Job drawing, mm, ordinate dimensions from the low corner. One solid piece. A direction names the side the tool comes from. Round coordinates to 2 decimals unless told otherwise and drop trailing zeros. Loops run counter-clockwise (first coordinate to the right, second up) from the corner with the lowest first, then second, coordinate; pieces in that order, holes last. Notation, with made-up numbers: M 70.5,69.5 L 119.5,69.5 A22 ccw 119.5,84.5 Z; hole C 63.5,19.5 d7. An arc over 180 degrees is marked long. Use a Markdown table: item, result. Add a question column.
(1) Band-saw the part on B-B, the plane z = 68. Write the cut outline in (x, y).
(2) Which spindle directions (+Z, -Z, +X, -X, +Y, -Y) get a long thin tool onto all of the face, cutting with end or side? Do the marked faces 3 and 4. Say none if no direction does.
(3) Band-saw the part on C-C, the plane x = 40. Write the cut outline in (y, z).
(4) Wall check: L1, parallel to Z at x = 75, y = 7.75; L2, parallel to X at y = 8.5, z = 6 (1 decimal). Give the ranges that are in metal, low to high.
(5) Flat gauge pins, fed straight in: P1, Ø6, axis at x = 75, z = 75, coming from the -Y side; P2, Ø1, axis at y = 3.5, z = 13, coming from the +X side (1 decimal); P3, Ø12, axis at x = 12.5, z = 29, coming from the -Y side; P4, Ø4, axis at x = 60, y = 3.5, coming from the -Z side. Where does each tip first touch, or does it go through?
(6) Two-plate mould, pull along Z, no slides. Class the marked faces 1 and 2: released by +Z, released by -Z, zero draft, split by the parting line, or undercut.
(7) Band-saw the part on A-A, the plane y = 6.75. Write the cut outline in (x, z).
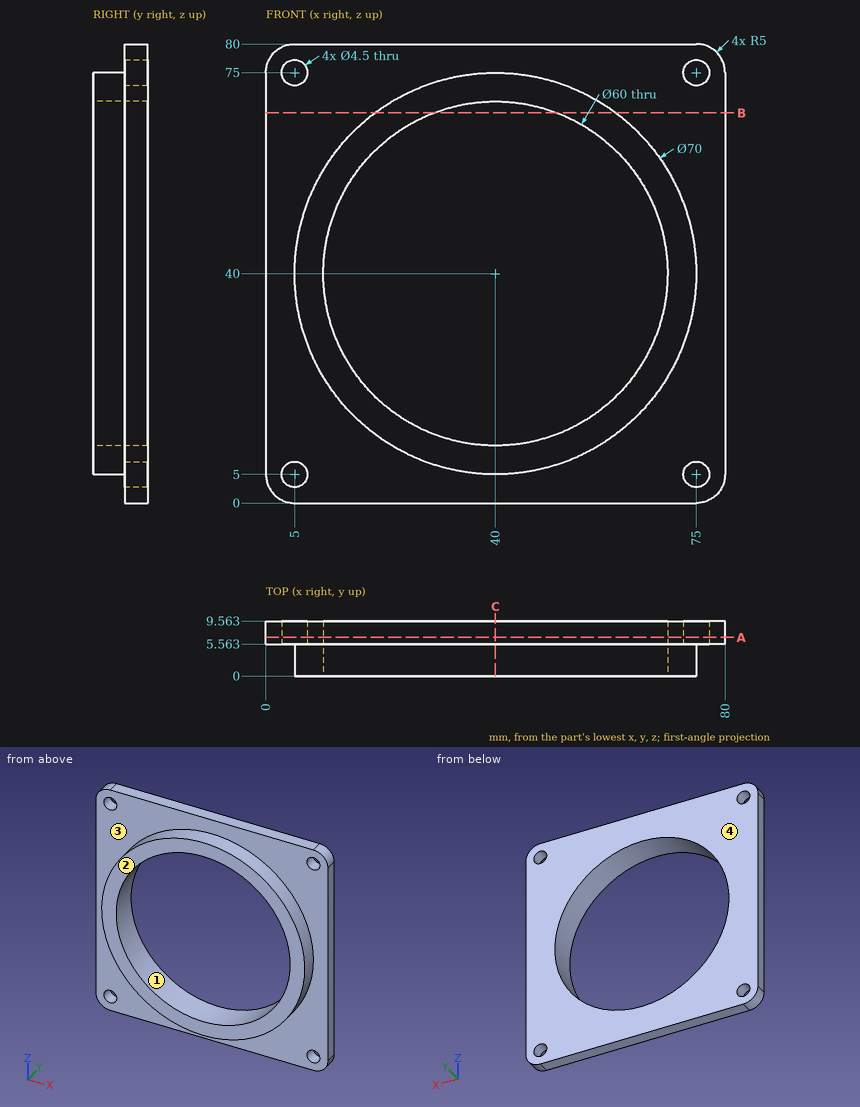
Return value:
| question | item | result |
|---|---|---|
| 1 | outline | M 0,5.56 L 19,5.56 L 19,0 L 29.23,0 L 29.23,9.56 L 0,9.56 Z; M 50.77,0 L 61,0 L 61,5.56 L 80,5.56 L 80,9.56 L 50.77,9.56 Z |
| 2 | face 3 | -Y |
| 2 | face 4 | +Z, -Z, +X, -X, +Y |
| 3 | outline | M 0,5 L 5.56,5 L 5.56,0 L 9.56,0 L 9.56,10 L 0,10 Z; M 0,70 L 9.56,70 L 9.56,80 L 5.56,80 L 5.56,75 L 0,75 Z |
| 4 | L1 | 0 to 2.75, 7.25 to 72.75, 77.25 to 80 |
| 4 | L2 | 0 to 3, 7 to 73, 77 to 80 |
| 5 | P1 | y = 5.56 |
| 5 | P2 | x = 62.9 |
| 5 | P3 | y = 0 |
| 5 | P4 | z = 9.98 |
| 6 | face 1 | undercut |
| 6 | face 2 | zero draft |
| 7 | outline | M 0,5 A5 ccw 5,0 L 75,0 A5 ccw 80,5 L 80,75 A5 ccw 75,80 L 5,80 A5 ccw 0,75 Z; hole C 5,5 d4.5; hole C 5,75 d4.5; hole C 40,40 d60; hole C 75,5 d4.5; hole C 75,75 d4.5 |
